The listing builds one solid part. Answer for the finished solid, in the listing's coordinates (mm). A direction names the side the tool comes from. Give positions to 0.01 mm unless a question says otherwise; leave off trailing zeros. Write each loop counter-clockwise with the first axis right and the second up, starting at its lowest first coordinate (ties: lowest second). Pieces come first, ordered by that corner, then holes. Notation, with made-up numbers: (43, 75) - (69, 75) arc R21 cw to (69, 84) - close; hole circle Ø1 at (75.5, 70). An arc over 180 degrees is marked (long way). One line per question, with ' | ' between items. Start each with the question number.
1. Find the intervals of material crossed by L1, parallel to X at y = 158.5, z = 7.75 (1 decimal); L2, parallel to X at y = 522, z = 5.75; L3, parallel to Y at x = -104, z = -7.75 (1 decimal), in increasing order. Write a range as from..to.
2. A cutting plane is placed at C-C (z = -2.25). Determine the outline of the cut face in (x, y) (1 decimal), then the cut area to 3 significant figures.
3. The mould has two halves that part along Y. Classify faces 1 (the face through (4, 593.725, 0)), 2 (the face through (-4, 4.762, 0)), 3 (the face through (-296.862, 301, 0)): +Y half, -Y half, draft (parallel to the pull), parting line (faces both ways), or undercut.
4. For faces 4 (the face through (-292.1, 301, 0)), 5 (the face through (-284, 320, -9.525)), determine the directions among +Z, -Z, +X, -X, +Y, -Y from which every point of the face is accessible in a straight line to the end or side of a thin tool.
```python
from build123d import *


with BuildPart() as part:
    # Sweep1: sweep along a path in Sketch2
    with BuildLine(Plane.XY) as sweep1_path:
        Line((-296.8625, 593.725), (296.8625, 593.725))
        Line((296.8625, 593.725), (296.8625, 0))
        Line((296.8625, 0), (-296.8625, 0))
        Line((-296.8625, 0), (-296.8625, 593.725))
    # Sketch1 → Sweep1 (sweep)
    with BuildSketch(Plane(origin=(0, 0, 0), x_dir=(0, 0, -1), z_dir=(1, 0, 0))):
        Polygon((-9.525, 14.2875), (-9.525, 0), (9.525, 0), (9.525, 14.2875), (6.35, 14.2875), (6.35, 4.7625), (-6.35, 4.7625), (-6.35, 14.2875), align=None)
    sweep(path=sweep1_path.line, transition=Transition.RIGHT)


solid = part.part
```
Determined:
1) L1: -296.9..-282.6, 282.6..296.9 | L2: -296.86..-292.1, 292.1..296.86 | L3: 0..14.3, 579.4..593.7
2) outline: (-296.9, 0) - (296.9, 0) - (296.9, 593.7) - (-296.9, 593.7) - close; hole (-292.1, 4.8) - (292.1, 4.8) - (292.1, 589) - (-292.1, 589) - close | area: 11,200 mm2
3) face 1: +Y half | face 2: undercut | face 3: draft
4) face 4: none | face 5: -Z, +X, -X, +Y, -Y
